Can you work these out from the model? Positions are in its coordinate system, mm. Coordinates: 2 decimals unless noted, no trailing zeros. Order: outer loops, then holes, each group sorted by start corner. A loop starts at its lowest first (then second) coordinate and runs counter-clockwise, first axis right, second up. Notation, with made-up numbers: (4.5, 75.5) -> (37.5, 75.5) arc R18 ccw to (37.5, 89.5) -> close; hole circle Ø1 at (89, 62.5). An arc over 180 degrees is marked (long way). Answer in a Markdown table with one row per item. Add a question column.
1. If I drill on line 1 along Y through (x, z) = (29, -2.75); line 2 along X through (y, z) = (-82, -0.75); line 3 along X through (y, z) = (-81.5, -2), over which ranges is the centre line in solid material (lowest first)? Write a range as [from, to].
2. Will these pins go through, and if not, where does the flat tip stop? pin 1 (15 mm diameter, centred on x = 29, y = -29, fed in from -Z); pin 2 (1.5 mm diameter, centred on x = -21.5, y = -46.5, fed in from +Z).
3. Imagine slicing it at B-B on x = 76. Write out the boundary of the cut face in (y, z), plus the area to 3 significant figures.
4. Imagine slicing it at A-A on y = -29. Write out the boundary of the cut face in (x, z).
5. Imagine slicing it at C-C on z = -3.25. State how many separate pieces and enclosed holes the cut face has, plus the area to 3 significant figures.
6. Imagine slicing it at D-D on x = 33. Write out the boundary of the cut face in (y, z), plus the area to 3 significant figures.
Solid Edge part; units mm, degrees
sketch "Sketch1" plane through (0, 0, 0) normal (0, 0, 1) x (1, 0, 0)
  line L0 (105, -116) -> (0, -116)
  line L1 (-105, -116) -> (0, -116)
  line L2 (-105, 0) -> (-105, -116)
  line L3 (0, 0) -> (-105, 0)
  line L4 (0, 0) -> (105, 0)
  line L5 (105, 0) -> (105, -116)
extrude "Protrusion1" add sketch "Sketch1" against normal blind 8
sketch "Sketch2" plane through (0, -58, 0) normal (0, 0, 1) x (1, 0, 0)
  circle A0 centre (-29, 29) radius 9.5
extrude "ExtrudedCutout_2" cut sketch "Sketch2" against normal blind 8
pattern_linear "Pattern1" count 2 spacing 47 along (-1, 0, 0) count 2 spacing 58 along (0, -1, 0) of "ExtrudedCutout_2"
mirror "Mirror1" about plane through (0, -58, -4) normal (-1, 0, 0) of "ExtrudedCutout_2", "Pattern1"
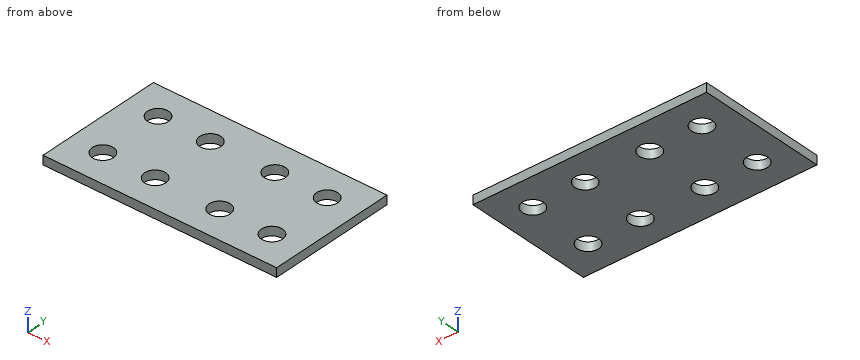
Answers follow:
| question | item | result |
|---|---|---|
| 1 | line 1 | y = [-116, -96.5], [-77.5, -38.5], [-19.5, 0] |
| 1 | line 2 | x = [-105, -84.08], [-67.92, -37.08], [-20.92, 20.92], [37.08, 67.92], [84.08, 105] |
| 1 | line 3 | x = [-105, -83.75], [-68.25, -36.75], [-21.25, 21.25], [36.75, 68.25], [83.75, 105] |
| 2 | pin 1 | passes through |
| 2 | pin 2 | stops at z = 0 |
| 3 | outline | (-116, -8) -> (-96.5, -8) -> (-96.5, 0) -> (-116, 0) -> close; (-77.5, -8) -> (-38.5, -8) -> (-38.5, 0) -> (-77.5, 0) -> close; (-19.5, -8) -> (0, -8) -> (0, 0) -> (-19.5, 0) -> close |
| 3 | area | 624 mm² |
| 4 | outline | (-105, -8) -> (-85.5, -8) -> (-85.5, 0) -> (-105, 0) -> close; (-66.5, -8) -> (-38.5, -8) -> (-38.5, 0) -> (-66.5, 0) -> close; (-19.5, -8) -> (19.5, -8) -> (19.5, 0) -> (-19.5, 0) -> close; (38.5, -8) -> (66.5, -8) -> (66.5, 0) -> (38.5, 0) -> close; (85.5, -8) -> (105, -8) -> (105, 0) -> (85.5, 0) -> close |
| 5 | separate pieces | 1 |
| 5 | enclosed holes | 8 |
| 5 | area | 22,100 mm² |
| 6 | outline | (-116, -8) -> (-95.62, -8) -> (-95.62, 0) -> (-116, 0) -> close; (-78.38, -8) -> (-37.62, -8) -> (-37.62, 0) -> (-78.38, 0) -> close; (-20.38, -8) -> (0, -8) -> (0, 0) -> (-20.38, 0) -> close |
| 6 | area | 652 mm² |
